Verification items for the finished model (mm, model axes). A direction names the side the tool comes from. Give positions to 0.01 mm unless a question says otherwise; leave off trailing zeros. Write each loop counter-clockwise with the first axis right and the second up, starting at its lowest first coordinate (ties: lowest second). Pieces come first, ordered by that corner, then holes. Notation, with made-up numbers: M 37,-18.75 L 83,-18.75 A4 cw 83,-13.75 Z; hole C 56,20.25 d1. An arc over 180 degrees is marked long. Write item = value, one per line.
from build123d import *

# Parameters (mm, degrees)
SKETCH2_W          = 178
SKETCH2_H          = 282
BASE_FLANGE1_DEPTH = 10
EDGE_FLANGE2_DEPTH = 282


# Sheet-metal steps are written as plain solids
with BuildPart() as part:
    # Sketch2 → Base-Flange1 (new body)
    with BuildSketch(Plane.XY):
        Rectangle(SKETCH2_W, SKETCH2_H)
    extrude(amount=BASE_FLANGE1_DEPTH)

    # Edge-Flange2 section (across the edge) → Edge-Flange2 (add)
    with BuildSketch(Plane(origin=(-222.83029789, 141, 10), x_dir=(0.7660444431189746, 0, 0.6427876096865435), z_dir=(0, -1, 0))):
        with BuildLine():
            Line((-10, 133.83029789), (-10, 135.336923418))
            Line((-10, 135.336923418), (0, 135.336923418))
            Line((0, 135.336923418), (0, 133.83029789))
            ThreePointArc((0, 133.83029789), (26.88966512, 12.538856771), (102.51995602, -86.024457285))
            Line((102.51995602, -86.024457285), (96.092079923, -93.684901716))
            ThreePointArc((96.092079923, -93.684901716), (17.82658725, 8.312674153), (-10, 133.83029789))
        make_face()
    extrude(amount=EDGE_FLANGE2_DEPTH)


solid = part.part
1) Cross-section at A-A on y = 45. Record the boundary of the cut face in (x, z).
From the geometry:
outline = M -317.48,107.25 L -316.52,106.09 A297 ccw -89,0 L 89,0 L 89,10 L -89,10 A287 cw -308.85,112.52 L -309.82,113.67 Z
2) Tool access check on faces 1 (the flat face through (-109, 141, 10)), 2 (the flat face through (-1, 2, 10)). Record the directions out of +Z, -Z, +X, -X, +Y, -Y that give a thin tool (end or side, any length) a straight path to the whole face; none if there is none.
From the geometry:
face_1 = +Z, -Z, +X, -X, +Y
face_2 = +Z, +X, +Y, -Y
3) Cross-section at C-C on z = 89.5. Record the boundary of the cut face in (x, y).
From the geometry:
outline = M -301.49,-141 L -287.27,-141 L -287.27,141 L -301.49,141 Z
4) Cross-section at B-B on x = -77.5. Record the boundary of the cut face in (y, z), plus the area to 3 significant figures.
From the geometry:
outline = M -141,0 L 141,0 L 141,10 L -141,10 Z
area = 2,820 mm^2
5) Depth check by flat-ended pin: P1, Ø10, axis at x = -77.5, y = -59.5, coming from the +Z side; P2, Ø1.5, axis at y = -75.5, z = 86.5, coming from the +X side; P3, Ø10, axis at x = -267.5, z = 52.5, coming from the -Y side; P4, Ø1.5, axis at x = -120, y = -24.5, coming from the +Z side. Enter the tip coordinate at first touch or a pass-through.
From the geometry:
P1 = 10
P2 = -283.27
P3 = through
P4 = 11.76
6) Material ranges on probe 1 along Z at (x, y) = (14.5, -103); probe 2 along X at (y, z) = (48, 54); probe 3 along Z at (x, y) = (-194, -19.5), recorded low to high. Write a range as from..to.
From the geometry:
probe_1 = 0..10
probe_2 = -259.76..-241.71
probe_3 = 19.18..29.9
